Part print with two shaded views. Sizes in mm from the minimum x, y, z corner. Give positions to 0.01 mm unless a question says otherwise; leave off trailing zeros. Order: outer loops, then holes, each group sorted by start corner. A loop starts at its lowest first (then second) coordinate and runs counter-clockwise, first axis right, second up. Notation, with made-up numbers: M -23,63 L -4,63 A24 ccw -4,96 Z; hole C 15,-36.75 d3. An arc over 180 degrees is marked long. Answer as CSV lines item,"result".
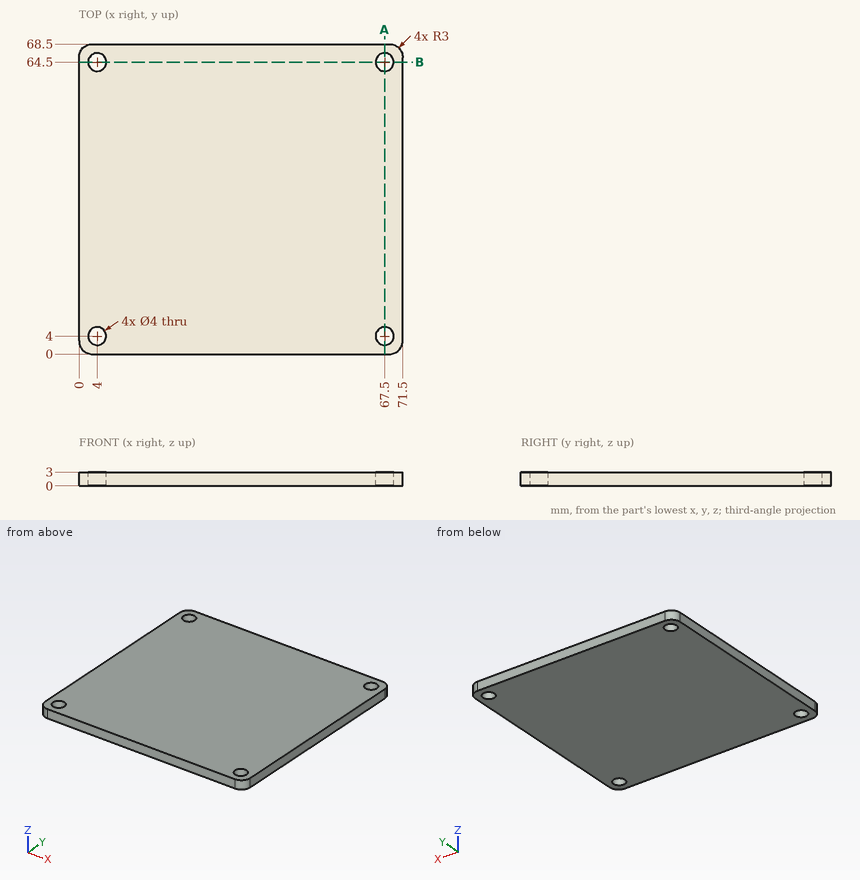
Item 1: Probe line 1 along Y through (x, z) = (67.5, 0.7); line 2 along Y through (x, z) = (4.5, 2.85). List the from-to ranges inside material, lowest first. Write a range as from..to.
Geometry says:
line 1,"y = 0..2, 6..62.5, 66.5..68.5"
line 2,"y = 0..2.06, 5.94..62.56, 66.44..68.5"
Item 2: Band-saw the part on B-B (y = 64.5). Give the cut face in (x, z).
Geometry says:
outline,"M 0,0 L 2,0 L 2,3 L 0,3 Z; M 6,0 L 65.5,0 L 65.5,3 L 6,3 Z; M 69.5,0 L 71.5,0 L 71.5,3 L 69.5,3 Z"
Item 3: Drop a flat-ended pin along its axis: pin 1 (2.5 mm diameter, centred on x = 67.5, y = 4, fed in from +Z). Give the stop position or say it passes through.
Geometry says:
pin 1,"passes through"
Item 4: Band-saw the part on A-A (x = 67.5). Give the cut face in (y, z).
Geometry says:
outline,"M 0,0 L 2,0 L 2,3 L 0,3 Z; M 6,0 L 62.5,0 L 62.5,3 L 6,3 Z; M 66.5,0 L 68.5,0 L 68.5,3 L 66.5,3 Z"
